from build123d import *

# Parameters (mm, degrees)
F0_W         = 60.96
F0_H         = 104.14
F0_R         = 17.78
F0_W_2       = 50.8
F0_H_2       = 38.1
F0_R_2       = 7.62
F5_DEPTH     = 12.7
F6_R         = 5.08
F7_R         = 1.27
F8_T1_DEPTH  = 7.62
F8_T4_ANGLE  = 90
F8_S7_W      = 5.08
F8_S7_H      = 5.08
F8_T8_DEPTH  = 5.08
F9_T1_DEPTH  = 7.62
F9_T4_ANGLE  = 90
F9_S7_W      = 5.08
F9_S7_H      = 5.08
F9_T8_DEPTH  = 5.08
F10_T1_DEPTH = 7.62
F10_T4_ANGLE = 90
F10_S7_W     = 5.08
F10_S7_H     = 5.08
F10_T8_DEPTH = 5.08
F11_T1_DEPTH = 7.62
F11_T4_ANGLE = 90
F11_S7_W     = 5.08
F11_S7_H     = 5.08
F11_T8_DEPTH = 5.08
F3_W         = 25.4
F3_H         = 2.54
F12_DEPTH    = 5.08
F4_W         = 9.1439969838
F4_H         = 2.7940007858
F13_DEPTH    = 1.27
F4_R         = 1.8751327249
F14_DEPTH    = 12.7
F17_DEPTH    = 0.508


# Not quite as in the source:
# - a fillet or chamfer that OpenCascade refuses, or shapes differently, is made with other operations: its cross-section is extruded or revolved along the edge and cut away or added


with BuildPart() as f5:
    # F0 (on Top) → F5 (new body)
    with BuildSketch(Plane.XY):
        Rectangle(F0_W, F0_H)
        with Locations((0, -21.59)):
            Circle(F0_R, mode=Mode.SUBTRACT)
        with Locations((0, 26.67)):
            Rectangle(F0_W_2, F0_H_2, mode=Mode.SUBTRACT)
        with Locations((0, 26.67)):
            Rectangle(F0_W_2, F0_H_2)
        with Locations((0, -21.59)):
            Circle(F0_R)
        with Locations((0, -21.59)):
            Circle(F0_R_2, mode=Mode.SUBTRACT)
        with Locations((0, -21.59)):
            Circle(F0_R_2)
    extrude(amount=-F5_DEPTH)

    # F6
    f6_edges = [f5.edges().sort_by_distance(p)[0] for p in [
        (0, -52.07, -12.7),
        (30.48, 0, -12.7),
        (0, 52.07, -12.7),
        (-30.48, 0, -12.7),
    ]]
    fillet(f6_edges, radius=F6_R)

    # F7
    f7_edges = [f5.edges().sort_by_distance(p)[0] for p in [
        (0, -52.07, 0),
        (30.48, 0, 0),
        (0, 52.07, 0),
        (-30.48, 0, 0),
    ]]
    fillet(f7_edges, radius=F7_R)

    # F8: fillet of radius 5.08 on 3 edges, made by hand

    # F8_s2 → F8_t1 (cut)
    with BuildSketch(Plane.XY.offset(-7.62)):
        with BuildLine():
            ThreePointArc((-25.4, -52.07), (-28.9921024484, -50.5821024484), (-30.48, -46.99))
            Line((-30.48, -46.99), (-30.48, -52.07))
            Line((-30.48, -52.07), (-25.4, -52.07))
        make_face()
    extrude(amount=F8_T1_DEPTH, mode=Mode.SUBTRACT)

    # F8_s3 → F8_t4 (revolve, cut)
    with BuildSketch(Plane.XZ.offset(46.99)):
        with BuildLine():
            ThreePointArc((-29.21, 0), (-30.1080256121, -0.3719743879), (-30.48, -1.27))
            Line((-30.48, -1.27), (-30.48, 0))
            Line((-30.48, 0), (-29.21, 0))
        make_face()
    revolve(axis=Axis((-25.4, -46.99, 0), (0, 0, 1)), revolution_arc=F8_T4_ANGLE, mode=Mode.SUBTRACT)


with BuildPart() as f8_tool6:
    # F8_s7 → F8_t8 (new body)
    with BuildSketch(Plane.XZ.offset(46.99)):
        with Locations((-27.94, -10.16)):
            Rectangle(F8_S7_W, F8_S7_H)
    extrude(amount=F8_T8_DEPTH)

    # F8_s9 → F8_t10 (revolve, cut)
    with BuildSketch(Plane(origin=(-25.4, -46.99, -7.62), x_dir=(0.7071067812, 0, 0.7071067812), z_dir=(0.7071067812, 0, -0.7071067812))):
        with BuildLine():
            ThreePointArc((0, -5.08), (5.08, 0), (0, 5.08))
            Line((0, 5.08), (0, -5.08))
        make_face()
    revolve(axis=Axis((-25.4, -46.99, -7.62), (0, -1, 0)), mode=Mode.SUBTRACT)


with BuildPart() as f5_1:
    add(f5.part)

    # F8_t5: cut F8_tool6
    add(f8_tool6.part, mode=Mode.SUBTRACT)

    # F9: fillet of radius 5.08 on 3 edges, made by hand

    # F9_s2 → F9_t1 (cut)
    with BuildSketch(Plane.XY.offset(-7.62)):
        with BuildLine():
            ThreePointArc((25.4, -52.07), (28.9921024484, -50.5821024484), (30.48, -46.99))
            Line((30.48, -46.99), (30.48, -52.07))
            Line((30.48, -52.07), (25.4, -52.07))
        make_face()
    extrude(amount=F9_T1_DEPTH, mode=Mode.SUBTRACT)

    # F9_s3 → F9_t4 (revolve, cut)
    with BuildSketch(Plane.YZ.offset(25.4)):
        with BuildLine():
            ThreePointArc((-50.8, 0), (-51.6980256121, -0.3719743879), (-52.07, -1.27))
            Line((-52.07, -1.27), (-52.07, 0))
            Line((-52.07, 0), (-50.8, 0))
        make_face()
    revolve(axis=Axis((25.4, -46.99, 0), (0, 0, 1)), revolution_arc=F9_T4_ANGLE, mode=Mode.SUBTRACT)


with BuildPart() as f9_tool6:
    # F9_s7 → F9_t8 (new body)
    with BuildSketch(Plane.XZ.offset(46.99)):
        with Locations((27.94, -10.16)):
            Rectangle(F9_S7_W, F9_S7_H)
    extrude(amount=F9_T8_DEPTH)

    # F9_s9 → F9_t10 (revolve, cut)
    with BuildSketch(Plane(origin=(25.4, -46.99, -7.62), x_dir=(-0.7071067812, 0, 0.7071067812), z_dir=(0.7071067812, 0, 0.7071067812))):
        with BuildLine():
            ThreePointArc((0, -5.08), (5.08, 0), (0, 5.08))
            Line((0, 5.08), (0, -5.08))
        make_face()
    revolve(axis=Axis((25.4, -46.99, -7.62), (0, -1, 0)), mode=Mode.SUBTRACT)


with BuildPart() as f5_2:
    add(f5_1.part)

    # F9_t5: cut F9_tool6
    add(f9_tool6.part, mode=Mode.SUBTRACT)

    # F10: fillet of radius 5.08 on 3 edges, made by hand

    # F10_s2 → F10_t1 (cut)
    with BuildSketch(Plane.XY.offset(-7.62)):
        with BuildLine():
            ThreePointArc((30.48, 46.99), (28.9921024484, 50.5821024484), (25.4, 52.07))
            Line((25.4, 52.07), (30.48, 52.07))
            Line((30.48, 52.07), (30.48, 46.99))
        make_face()
    extrude(amount=F10_T1_DEPTH, mode=Mode.SUBTRACT)

    # F10_s3 → F10_t4 (revolve, cut)
    with BuildSketch(Plane.XZ.offset(-46.99)):
        with BuildLine():
            ThreePointArc((29.21, 0), (30.1080256121, -0.3719743879), (30.48, -1.27))
            Line((30.48, -1.27), (30.48, 0))
            Line((30.48, 0), (29.21, 0))
        make_face()
    revolve(axis=Axis((25.4, 46.99, 0), (0, 0, 1)), revolution_arc=F10_T4_ANGLE, mode=Mode.SUBTRACT)


with BuildPart() as f10_tool6:
    # F10_s7 → F10_t8 (new body)
    with BuildSketch(Plane.YZ.offset(25.4)):
        with Locations((49.53, -10.16)):
            Rectangle(F10_S7_W, F10_S7_H)
    extrude(amount=F10_T8_DEPTH)

    # F10_s9 → F10_t10 (revolve, cut)
    with BuildSketch(Plane(origin=(25.4, 46.99, -7.62), x_dir=(0, -0.7071067812, 0.7071067812), z_dir=(0, 0.7071067812, 0.7071067812))):
        with BuildLine():
            ThreePointArc((0, -5.08), (5.08, 0), (0, 5.08))
            Line((0, 5.08), (0, -5.08))
        make_face()
    revolve(axis=Axis((25.4, 46.99, -7.62), (1, 0, 0)), mode=Mode.SUBTRACT)


with BuildPart() as f5_3:
    add(f5_2.part)

    # F10_t5: cut F10_tool6
    add(f10_tool6.part, mode=Mode.SUBTRACT)

    # F11: fillet of radius 5.08 on 3 edges, made by hand

    # F11_s2 → F11_t1 (cut)
    with BuildSketch(Plane.XY.offset(-7.62)):
        with BuildLine():
            ThreePointArc((-30.48, 46.99), (-28.9921024484, 50.5821024484), (-25.4, 52.07))
            Line((-25.4, 52.07), (-30.48, 52.07))
            Line((-30.48, 52.07), (-30.48, 46.99))
        make_face()
    extrude(amount=F11_T1_DEPTH, mode=Mode.SUBTRACT)

    # F11_s3 → F11_t4 (revolve, cut)
    with BuildSketch(Plane.YZ.offset(-25.4)):
        with BuildLine():
            ThreePointArc((50.8, 0), (51.6980256121, -0.3719743879), (52.07, -1.27))
            Line((52.07, -1.27), (52.07, 0))
            Line((52.07, 0), (50.8, 0))
        make_face()
    revolve(axis=Axis((-25.4, 46.99, 0), (0, 0, 1)), revolution_arc=F11_T4_ANGLE, mode=Mode.SUBTRACT)


with BuildPart() as f11_tool6:
    # F11_s7 → F11_t8 (new body)
    with BuildSketch(Plane.YZ.offset(-25.4)):
        with Locations((49.53, -10.16)):
            Rectangle(F11_S7_W, F11_S7_H)
    extrude(amount=-F11_T8_DEPTH)

    # F11_s9 → F11_t10 (revolve, cut)
    with BuildSketch(Plane(origin=(-25.4, 46.99, -7.62), x_dir=(0, -0.7071067812, 0.7071067812), z_dir=(0, -0.7071067812, -0.7071067812))):
        with BuildLine():
            ThreePointArc((0, -5.08), (5.08, 0), (0, 5.08))
            Line((0, 5.08), (0, -5.08))
        make_face()
    revolve(axis=Axis((-25.4, 46.99, -7.62), (-1, 0, 0)), mode=Mode.SUBTRACT)


with BuildPart() as f5_4:
    add(f5_3.part)

    # F11_t5: cut F11_tool6
    add(f11_tool6.part, mode=Mode.SUBTRACT)

    # F3 (on line) → F12 (cut)
    with BuildSketch(Plane.XZ.offset(52.07)):
        with Locations((0, -3.81)):
            Rectangle(F3_W, F3_H)
    extrude(amount=-F12_DEPTH, mode=Mode.SUBTRACT)

    # F4 (on line) → F13 (cut)
    with BuildSketch(Plane.XZ.offset(-52.07)):
        with Locations((-20.4787496477, -3.7782501895)):
            Rectangle(F4_W, F4_H)
    extrude(amount=F13_DEPTH, mode=Mode.SUBTRACT)

    # F4 (on line) → F14 (cut)
    with BuildSketch(Plane.XZ.offset(-52.07)):
        with Locations((17.7482496947, -3.5242501181)):
            Circle(F4_R)
        with Locations((-20.4787496477, -3.7782501895)):
            Rectangle(F4_W, F4_H)
    extrude(amount=F14_DEPTH, mode=Mode.SUBTRACT)

    # F15 (on Right) → F16 (revolve, cut)
    with BuildSketch(Plane.YZ):
        Polygon((-20.5422501868, 5.2387503395), (-38.3222501868, 4.4979169496), (-38.3222501868, -0.1322916101), (-28.1622501868, -2.54), (-20.5422501868, -2.54), align=None)
    revolve(axis=Axis((0, -20.5422501868, 1.3493751698), (0, 0, 1)), mode=Mode.SUBTRACT)

    # F0 (on Top) → F17 (cut)
    with BuildSketch(Plane.XY):
        with Locations((0, 26.67)):
            Rectangle(F0_W_2, F0_H_2)
    extrude(amount=-F17_DEPTH, mode=Mode.SUBTRACT)


solid = f5_4.part
Could you check a few things on this model? Use its own coordinates, in mm. A direction names the side the tool comes from. Round coordinates to 2 decimals unless told otherwise and drop trailing zeros. Write each loop counter-clockwise with the first axis right and the second up, starting at its lowest first coordinate (ties: lowest second). Pieces come first, ordered by that corner, then holes. Notation, with made-up numbers: (-17, 85) - (37, 85) arc R18 ccw to (37, 89) - close; hole circle Ø11 at (29, 67). An arc over 180 degrees is marked (long way). Use a Markdown table: item, result.
Q1. Please list where these lines run through material, in increasing order: L1, parallel to Z at x = -17, y = 27; L2, parallel to X at y = -41.5, z = -11; L3, parallel to X at y = -26.5, z = -8.
Output values:
| item | result |
|---|---|
| L1 | -12.7 to -0.51 |
| L2 | -29.19 to 29.19 |
| L3 | -30.47 to 30.47 |
Q2. I want a section at A-A (x = 0). List the corners of the cut face in (y, z) for me.
Output values:
| item | result |
|---|---|
| outline | (-52.07, -7.62) arc R5.08 ccw to (-46.99, -12.7) - (46.99, -12.7) arc R5.08 ccw to (52.07, -7.62) - (52.07, -1.27) arc R1.27 ccw to (50.8, 0) - (45.72, 0) - (45.72, -0.51) - (7.62, -0.51) - (7.62, 0) - (-2.76, 0) - (-2.76, -0.13) - (-12.92, -2.54) - (-28.16, -2.54) - (-38.32, -0.13) - (-38.32, 0) - (-50.8, 0) arc R1.27 ccw to (-52.07, -1.27) - (-52.07, -2.54) - (-46.99, -2.54) - (-46.99, -5.08) - (-52.07, -5.08) - close |
Q3. Thinking about a two-plate mould opening in X: for faces 4 (the flat face through (-21, 46, -2.381)), 5 (the cylindrical face through (29.031, 0.658, -11.172)), 6 (the cylindrical face through (-28.952, -50.621, -4.489)), which applies, released by +X, released by -X, zero draft, split by the parting line, or undercut?
Output values:
| item | result |
|---|---|
| face 4 | undercut |
| face 5 | released by +X |
| face 6 | released by -X |
Q4. For pin 1 (5 mm diameter, centred on y = -19, z = -11, fed in from -X); pin 2 (1.3 mm diameter, centred on y = -49.5, z = -4, fed in from +X); pin 3 (10 mm diameter, centred on x = -4, y = 40.5, fed in from +Z), each with a flat end and sliding along its axis, tell me the tip position at first contact or that it passes through.
Output values:
| item | result |
|---|---|
| pin 1 | x = -30.4 |
| pin 2 | x = 30.13 |
| pin 3 | z = -0.51 |
Q5. For faces 1 (the conical face through (0.357, -12.437, -2.423)), 2 (the flat face through (-21, 39.37, -4)), 3 (the flat face through (0, -50, -5.08)), which set-ups out of +Z, -Z, +X, -X, +Y, -Y let a thin tool reach every point of the face, with its end or its side?
Output values:
| item | result |
|---|---|
| face 1 | +Z |
| face 2 | +Y |
| face 3 | -Y |
Q6. I want a section at B-B (y = 12). List the corners of the cut face in (x, z) for me.
Output values:
| item | result |
|---|---|
| outline | (-30.48, -7.62) arc R5.08 ccw to (-25.4, -12.7) - (25.4, -12.7) arc R5.08 ccw to (30.48, -7.62) - (30.48, -1.27) arc R1.27 ccw to (29.21, 0) - (25.4, 0) - (25.4, -0.51) - (-25.4, -0.51) - (-25.4, 0) - (-29.21, 0) arc R1.27 ccw to (-30.48, -1.27) - close |
